For this review, take the finished solid that the model builds, in its own axes (mm). Coordinates: 2 decimals unless noted, no trailing zeros. Write each loop counter-clockwise with the first axis right and the second up, starting at its lowest first coordinate (ties: lowest second). Pieces come first, ordered by that corner, then holes. Notation, with made-up numbers: (64, -26) - (119, -26) arc R21 ccw to (119, 12) - close; hole circle Ø4 at (56, 88.5). An arc over 180 degrees is marked (long way). Use one line per item in the form item = value. Start each with the question number.
1) We need section C-C (x = -34.5). Give the boundary of the cut face in (y, z).
2) For L1, parallel to Z at x = -74, y = 19.5; L2, parallel to X at y = -27, z = 14.5; L3, parallel to Y at x = -88.5, z = 8.25, list the stretches that pass through material, from the lowest coordinate up. Write a range as from..to.
3) We need section A-A (y = -28). Give the boundary of the cut face in (x, z).
4) Insertion check: P1, Ø4, axis at x = -35, z = 11, coming from the -Y side; P2, Ø1, axis at x = -74, y = 29, coming from the -Z side; P3, Ø2, axis at x = -49.5, z = 8, coming from the +Y side; P4, Ø6, axis at x = -71, z = 10.5, coming from the +Y side. Each pin has a flat end and moves straight along its axis. Give the tip position at first contact, or say it passes through.
```python
from build123d import *

# Parameters (mm, degrees)
F1_DEPTH       = 25.4
F3_T           = -2.54
F4_D           = 6.35
F4_DEPTH       = 12.7
F4_CSINK_D     = 12.7
F4_CSINK_ANGLE = 90


with BuildPart() as f1:
    # F0 (on Top) → F1 (new body)
    with BuildSketch(Plane.XY):
        Polygon((95.277585, 49.860638), (-113.311097, 50.922569), (-113.311097, -73.111692), (-104.497745, -73.111692), (95.277585, -74.128754), align=None)
    extrude(amount=F1_DEPTH)

    # F3
    f3_openings = [f1.faces().sort_by_distance(p)[0] for p in [
        (95.277585, -12.134058, 12.7),
    ]]
    offset(amount=F3_T, openings=f3_openings)

    # F4
    with Locations(Plane(origin=(-113.311097, 0, 0), x_dir=(0, -1, 0), z_dir=(-1, 0, 0))):
        with Locations((-30.990601, 16.404929)):
            CounterSinkHole(F4_D / 2, F4_CSINK_D / 2, depth=F4_DEPTH, counter_sink_angle=F4_CSINK_ANGLE)


solid = f1.part
```
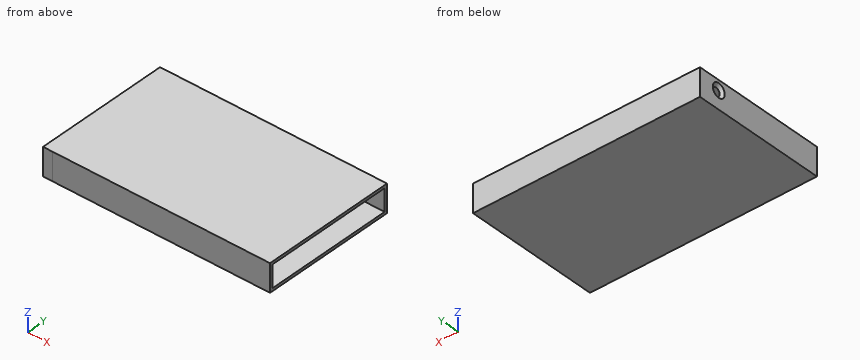
Determined:
q1.outline = (-73.47, 0) - (50.52, 0) - (50.52, 25.4) - (-73.47, 25.4) - close; hole (-70.93, 2.54) - (47.98, 2.54) - (47.98, 22.86) - (-70.93, 22.86) - close
q2.L1 = 0..2.54, 22.86..25.4
q2.L2 = -113.31..-110.77
q2.L3 = -73.19..-70.65, 48.26..50.8
q3.outline = (-113.31, 0) - (95.28, 0) - (95.28, 2.54) - (-110.77, 2.54) - (-110.77, 22.86) - (95.28, 22.86) - (95.28, 25.4) - (-113.31, 25.4) - close
q4.P1 = -73.48
q4.P2 = 0
q4.P3 = 50.6
q4.P4 = 50.72
